Input: dimensioned drawing with shaded views. Units: mm. Origin: part minimum x, y, z. A direction names the side the tool comes from. Coordinates: 2 decimals unless noted, no trailing zeros. Loops run counter-clockwise (first coordinate to the right, second up) from the corner with the lowest first, then second, coordinate; pieces in that order, holes last.
Item 1: Pull-direction query (Z, two-part tool) for the marked faces 3, 4 and 5; classes: +Z half, -Z half, draft (parallel to the pull), parting line (faces both ways), or undercut.
Item 2: Section query D-D, the plane x = 30.5. Return the cut outline in (y, z).
Item 3: Reachability of the marked faces 1 and 2 from +Z, -Z, +X, -X, +Y, -Y: full face, straight path, thin tool, end or side. Return the list, or none.
Item 4: Section query A-A, the plane x = 40. Return the cut outline in (y, z), then the cut area to 3 significant figures.
Item 5: Section query C-C, the plane z = 25.4. Return the cut outline in (x, y).
Item 6: Pin query (flat end, axial travel): pin 1 Ø5 at (x, y) = (52.5, 21.5) entering from +Z; pin 2 Ø1.5 at (y, z) = (10.5, 13) entering from -X; pin 3 Ø2 at (x, y) = (11.5, 7) entering from +Z. Return the tip coordinate at first contact, or that it passes through.
Item 7: Section query B-B, the plane y = 19.25. Return the cut outline in (x, z).
Item 8: Line query: probe 1 along Z at (x, y) = (40, 3.5); probe 2 along Z at (x, y) = (36, 8); probe 3 along X at (y, z) = (5.5, 34.5). Output: solid intervals per line, ascending.
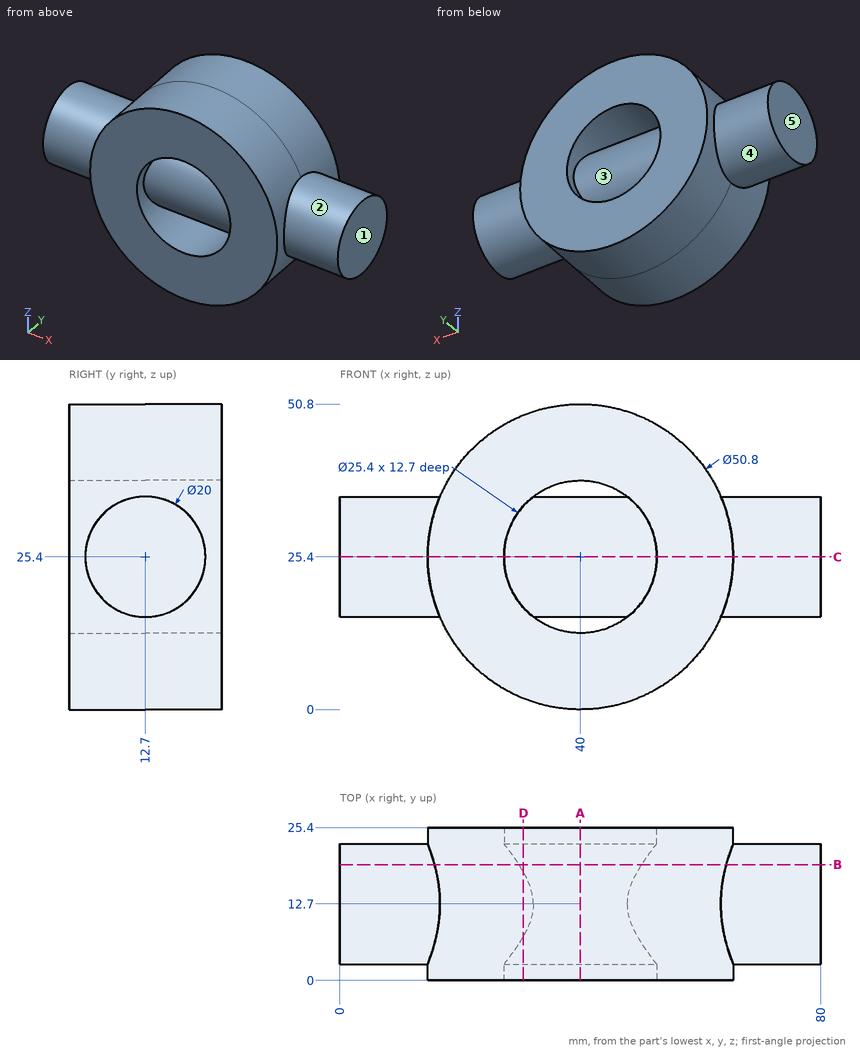
Verdict:
1. face 3: undercut
1. face 4: parting line
1. face 5: draft
2. outline: (0, 1.84) - (25.4, 1.84) - (25.4, 16.97) - (18.08, 16.97) arc R10 ccw to (18.08, 33.83) - (25.4, 33.83) - (25.4, 48.96) - (0, 48.96) - (0, 33.83) - (7.32, 33.83) arc R10 ccw to (7.32, 16.97) - (0, 16.97) - close
3. face 1: +Z, -Z, +X, +Y, -Y
3. face 2: +X
4. outline: (0, 0) - (25.4, 0) - (25.4, 12.7) - (0, 12.7) - close; (0, 38.1) - (25.4, 38.1) - (25.4, 50.8) - (0, 50.8) - close; circle Ø20 at (12.7, 25.4)
4. area: 959 mm2
5. outline: (0, 2.7) - (14.6, 2.7) - (14.6, 0) - (27.3, 0) - (27.3, 2.7) - (52.7, 2.7) - (52.7, 0) - (65.4, 0) - (65.4, 2.7) - (80, 2.7) - (80, 22.7) - (65.4, 22.7) - (65.4, 25.4) - (52.7, 25.4) - (52.7, 22.7) - (27.3, 22.7) - (27.3, 25.4) - (14.6, 25.4) - (14.6, 22.7) - (0, 22.7) - close
6. pin 1: stops at z = 48.75
6. pin 2: stops at x = 17.43
6. pin 3: stops at z = 34.23
7. outline: (0, 17.84) - (15.75, 17.84) arc R25.4 ccw to (64.25, 17.84) - (80, 17.84) - (80, 32.96) - (64.25, 32.96) arc R25.4 ccw to (15.75, 32.96) - (0, 32.96) - close; hole (29.79, 17.84) arc R12.7 ccw to (50.21, 17.84) - close; hole (29.79, 32.96) - (50.21, 32.96) arc R12.7 ccw to start
8. probe 1: z = 0 to 12.7, 21.48 to 29.32, 38.1 to 50.8
8. probe 2: z = 0.32 to 13.35, 16.57 to 34.23, 37.45 to 50.48
8. probe 3: x = 16.29 to 31.14, 48.86 to 63.71
